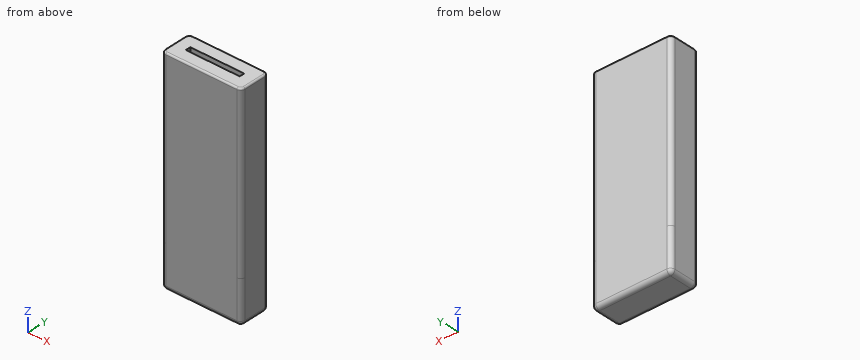
from build123d import *

# Parameters (mm, degrees)
F0_W     = 23.622
F0_H     = 9.144
F1_DEPTH = 12.7
F2_R     = 1.27
F3_W     = 16.002
F3_H     = 1.524
F4_DEPTH = 50.8
F5_R     = 0.508


with BuildPart() as f1:
    # F0 (on Top) → F1 (new body)
    with BuildSketch(Plane.XY):
        with Locations((-8.5595357362, -22.114415653)):
            Rectangle(F0_W, F0_H)
    extrude(amount=F1_DEPTH)

    # F2
    f2_edges = [f1.edges().sort_by_distance(p)[0] for p in [
        (-8.559536, -26.686416, 0),
        (-20.370536, -22.114416, 0),
        (-8.559536, -17.542416, 0),
        (3.251464, -22.114416, 0),
        (3.251464, -17.542416, 6.35),
        (-20.370536, -17.542416, 6.35),
        (-20.370536, -26.686416, 6.35),
        (3.251464, -26.686416, 6.35),
    ]]
    fillet(f2_edges, radius=F2_R)

    # F3 (on face) → F4 (join)
    with BuildSketch(Plane.XY.offset(12.7)):
        with BuildLine():
            ThreePointArc((3.2514642638, -18.812415653), (2.8794898759, -17.9143900409), (1.9814642638, -17.542415653))
            Line((1.9814642638, -17.542415653), (-19.1005357362, -17.542415653))
            ThreePointArc((-19.1005357362, -17.542415653), (-19.9985613483, -17.9143900409), (-20.3705357362, -18.812415653))
            Line((-20.3705357362, -18.812415653), (-20.3705357362, -25.416415653))
            ThreePointArc((-20.3705357362, -25.416415653), (-19.9985613483, -26.3144412652), (-19.1005357362, -26.686415653))
            Line((-19.1005357362, -26.686415653), (1.9814642638, -26.686415653))
            ThreePointArc((1.9814642638, -26.686415653), (2.8794898759, -26.3144412652), (3.2514642638, -25.416415653))
            Line((3.2514642638, -25.416415653), (3.2514642638, -18.812415653))
        make_face()
        with Locations((-8.5595357362, -22.114415653)):
            Rectangle(F3_W, F3_H, mode=Mode.SUBTRACT)
    extrude(amount=F4_DEPTH)

    # F5
    f5_edges = [f1.edges().sort_by_distance(p)[0] for p in [
        (-8.559536, -17.542416, 63.5),
        (3.251464, -22.114416, 63.5),
        (-8.559536, -26.686416, 63.5),
        (-20.370536, -22.114416, 63.5),
        (2.87949, -26.314441, 63.5),
        (-19.998561, -26.314441, 63.5),
        (-19.998561, -17.91439, 63.5),
        (2.87949, -17.91439, 63.5),
    ]]
    fillet(f5_edges, radius=F5_R)


solid = f1.part
Geometry check sheet. Reference: the model listing, model coordinates, mm. Round coordinates to 2 decimals unless told otherwise and drop trailing zeros. Loops run counter-clockwise (first coordinate to the right, second up) from the corner with the lowest first, then second, coordinate; pieces in that order, holes last.
Item 1: Thickness scan on line 1 (Y direction, x = -10, z = 24.5); line 2 (Z direction, x = -12, y = -22.25); line 3 (X direction, y = -22.5, z = 45.5). Record the ranges inside material, lowest first.
Item 2: Gauge pin test, flat end, axial feed: pin 1 (1.2 mm diameter, centred on x = -6, y = -22, fed in from +Z). Record the tip position at first contact, or that the pin passes through.
Item 3: Cross-section at A-A on z = 20.5. Record the boundary of the cut face in (x, y), then the cut area to 3 significant figures.
Item 4: Cross-section at B-B on x = -12.75. Record the boundary of the cut face in (y, z), then the cut area to 3 significant figures.
Answer sheet:
1. line 1: y = -26.69 to -22.88, -21.35 to -17.54
1. line 2: z = 0 to 12.7
1. line 3: x = -20.37 to -16.56, -0.56 to 3.25
2. pin 1: stops at z = 12.7
3. outline: (-20.37, -25.42) arc R1.27 ccw to (-19.1, -26.69) - (1.98, -26.69) arc R1.27 ccw to (3.25, -25.42) - (3.25, -18.81) arc R1.27 ccw to (1.98, -17.54) - (-19.1, -17.54) arc R1.27 ccw to (-20.37, -18.81) - close; hole (-16.56, -22.88) - (-0.56, -22.88) - (-0.56, -21.35) - (-16.56, -21.35) - close
3. area: 190 mm2
4. outline: (-26.69, 1.27) arc R1.27 ccw to (-25.42, 0) - (-18.81, 0) arc R1.27 ccw to (-17.54, 1.27) - (-17.54, 62.99) arc R0.51 ccw to (-18.05, 63.5) - (-21.35, 63.5) - (-21.35, 12.7) - (-22.88, 12.7) - (-22.88, 63.5) - (-26.18, 63.5) arc R0.51 ccw to (-26.69, 62.99) - close
4. area: 502 mm2
